Check sheet for the modelled part. Datum: model origin and axes. Units: mm. Face numbers are marked on the shaded views. Round coordinates to 2 decimals unless told otherwise and drop trailing zeros. Write each loop counter-clockwise with the first axis right and the second up, starting at its lowest first coordinate (ties: lowest second). Pieces come first, ordered by that corner, then holes.
Item 1: Release check for a two-part mould opening along X. For the marked faces 1, 2 and 3 record: pulls with the +X half, pulls with the -X half, needs draft (parallel to the pull), parting line crosses it, or undercut.
Item 2: Section check C-C, the plane z = 2.55. Record the cut outline in (x, y), plus the area to 3 significant figures.
Item 3: Depth check by flat-ended pin: pin 1 (2 mm diameter, centred on y = -0.5, z = 1.5, fed in from -X); pin 2 (1.5 mm diameter, centred on y = 6, z = 3, fed in from -X); pin 3 (1 mm diameter, centred on y = -3, z = 2.5, fed in from +X). Enter the tip coordinate at first touch or a pass-through.
Item 4: Material ranges on line 1 along X through (y, z) = (0.25, 2.1); line 2 along X through (y, z) = (5.75, 2.8), recorded low to high.
Item 5: Section check A-A, the plane x = 0. Record the cut outline in (y, z), plus the area to 3 significant figures.
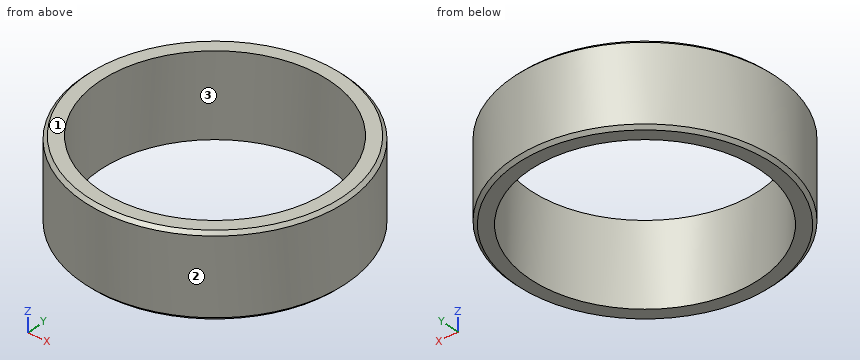
from build123d import *

# Parameters (mm, degrees)
CYLINDER002_R     = 7
CYLINDER002_DEPTH = 5
CYLINDER_R        = 8
CYLINDER_DEPTH    = 5
CHAMFER004_SIZE   = 0.2


with BuildPart() as cilindro:
    # Cylinder002 → Cylinder002 (new body)
    with BuildSketch(Plane.XY):
        Circle(CYLINDER002_R)
    extrude(amount=CYLINDER002_DEPTH)


with BuildPart() as exterior001:
    # Cylinder → Cylinder (new body)
    with BuildSketch(Plane.XY):
        Circle(CYLINDER_R)
    extrude(amount=CYLINDER_DEPTH)

    # Cut: cut Cilindro
    add(cilindro.part, mode=Mode.SUBTRACT)

    # Chamfer004
    chamfer004_edges = [exterior001.edges().sort_by_distance(p)[0] for p in [
        (-8, 0, 5),
        (-8, 0, 0),
    ]]
    chamfer(chamfer004_edges, length=CHAMFER004_SIZE)


solid = exterior001.part
Values found:
1. face 1: needs draft
1. face 2: parting line crosses it
1. face 3: undercut
2. outline: circle Ø16 at (0, 0); hole circle Ø14 at (0, 0)
2. area: 47.1 mm2
3. pin 1: stops at x = -8
3. pin 2: stops at x = -6.04
3. pin 3: stops at x = 7.6
4. line 1: x = -8 to -7, 7 to 8
4. line 2: x = -5.56 to -3.99, 3.99 to 5.56
5. outline: (-8, 0.2) - (-7.8, 0) - (-7, 0) - (-7, 5) - (-7.8, 5) - (-8, 4.8) - close; (7, 0) - (7.8, 0) - (8, 0.2) - (8, 4.8) - (7.8, 5) - (7, 5) - close
5. area: 9.92 mm2
